Autodesk Inventor part; units mm, degrees
ref_plane "YZ Plane" through (0, 0, 0) normal (1, 0, 0) x (0, 1, 0)
ref_plane "XZ Plane" through (0, 0, 0) normal (0, 1, 0) x (-1, 0, 0)
ref_plane "XY Plane" through (0, 0, 0) normal (0, 0, 1) x (1, 0, 0)
sketch "Эскиз1" plane through (0, 0, 0) normal (0, 1, 0) x (-1, 0, 0)
  circle A0 centre (0, 0) radius 42
  line L0 (0, -42) -> (0, 42) construction
  circle A1 centre (18.0767, -25) radius 9
  circle A2 centre (-18.0767, -25) radius 9
  line L1 (39.598, -14) -> (-39.598, -14)
  circle A3 centre (0, -30.8507) radius 9
  circle A4 centre (0, 0) radius 30.8507 construction
  line L2 (0, 0) -> (12.9332, -39.9591) construction
  line L3 (0, 0) -> (-12.9332, -39.9591) construction
  line L4 (9.9159, -38.7553) -> (14.673, -37.2156)
  line L5 (14.673, -37.2156) -> (15.2888, -39.1184)
  line L6 (15.2888, -39.1184) -> (10.5318, -40.6581)
  line L7 (10.5318, -40.6581) -> (9.9159, -38.7553)
  line L8 (9.9159, -38.7553) -> (15.2888, -39.1184) construction
  line L9 (14.673, -37.2156) -> (10.5318, -40.6581) construction
  line L10 (-14.673, -37.2156) -> (-9.9159, -38.7553)
  line L11 (-9.9159, -38.7553) -> (-10.5318, -40.6581)
  line L12 (-10.5318, -40.6581) -> (-15.2888, -39.1184)
  line L13 (-15.2888, -39.1184) -> (-14.673, -37.2156)
  line L14 (-14.673, -37.2156) -> (-10.5318, -40.6581) construction
  line L15 (-9.9159, -38.7553) -> (-15.2888, -39.1184) construction
  line L16 (-2.5, -16.8507) -> (2.5, -16.8507)
  line L17 (2.5, -16.8507) -> (2.5, -18.8507)
  line L18 (2.5, -18.8507) -> (-2.5, -18.8507)
  line L19 (-2.5, -18.8507) -> (-2.5, -16.8507)
  line L20 (-2.5, -16.8507) -> (2.5, -18.8507) construction
  line L21 (2.5, -16.8507) -> (-2.5, -18.8507) construction
  circle A5 centre (0, 0) radius 17.0352
  circle A6 centre (0, -44.5) radius 2.5
  circle A7 centre (0, 0) radius 50
  circle A8 centre (0, -44.5) radius 4
  circle A9 centre (-32, -19) radius 2.5
  circle A10 centre (32, -19) radius 2.5
  circle A11 centre (0, 0) radius 44 construction
  circle A12 centre (0, 2) radius 44
  circle A13 centre (31.1127, -29.1127) radius 2.5
  circle A14 centre (-31.1127, -29.1127) radius 2.5
  point P0 (12.6024, -38.9369)
  point P1 (-12.6024, -38.9369)
  point P2 (0, -17.8507)
  point P3 (9.7056, -14)
  point P4 (2.5, -16.8507)
  point P5 (-9.7056, -14)
  point P6 (-15.2888, -39.1184)
  point P7 (10.5318, -40.6581)
  point P8 (-3.0315, -41.8904)
  point P9 (3.0315, -41.8904)
  point P10 (0, -42)
  point P11 (28.9734, -30.4063)
  point P12 (32.2615, -26.8923)
  point P13 (-32.2615, -26.8923)
  point P14 (-28.9734, -30.4063)
  dimension "d0" = 84
  dimension "d5" = 18
  dimension "d7" = 14
  dimension "d8" = 11
  dimension "d13" = 35.87
  dimension "d14" = 17.935
  dimension "d15" = 2
  dimension "d16" = 2
  dimension "d17" = 5
  dimension "d18" = 5
  dimension "d19" = 5
  dimension "d20" = 2
  dimension "d21" = 13
  dimension "d27" = 100
  dimension "d28" = 5
  dimension "d29" = 8
  dimension "d30" = 5
  dimension "d31" = 19
  dimension "d32" = 64
  dimension "d34" = 19
  dimension "d35" = 88
  dimension "d37" = 2
  dimension "d38" = 88
  dimension "d39" = 5
  dimension "d40" = 90
extrude "Выдавливание2" add sketch "Эскиз1" along normal blind 3 contours L1 A5 L19 L18 L17 A0 A13 L5 L4 L7 A8 L11 L10 L13 A14 | A8 A0 A12 | A12 A0 A8 | A8 A0
fillet "Сопряжение3" radius 6 2 edges at (39.598, 1.5, -14) (-39.598, 1.5, -14)
fillet "Сопряжение4" radius 5 2 edges at (-32.2615, 1.5, -26.8923) (-28.9734, 1.5, -30.4063)
fillet "Сопряжение5" radius 5 2 edges at (28.9734, 1.5, -30.4063) (32.2615, 1.5, -26.8923)
equation "\"d14\" = 0.5 * d13"
properties part number "Крепление АКБ" material "Пластик АБС"
Check sheet for the modelled part. Datum: model origin and axes. Units: mm. A direction names the side the tool comes from. Round coordinates to 2 decimals unless told otherwise and drop trailing zeros. Loops run counter-clockwise (first coordinate to the right, second up) from the corner with the lowest first, then second, coordinate; pieces in that order, holes last. Notation, with made-up numbers: M -33,-20 L 16,-20 A17 cw 16,-4 Z; hole C -22,31 d10. An arc over 180 degrees is marked long. One line per item, written item: value.
(1) Sectioned sample at B-B, the plane z = -35.5. Record the cut outline in (x, y), then the cut area to 3 significant figures.
Computed values:
outline: M -22.44,0 L -7.71,0 L -7.71,3 L -22.44,3 Z; M 7.71,0 L 22.44,0 L 22.44,3 L 7.71,3 Z
area: 88.4 mm^2
(2) Sectioned sample at A-A, the plane x = 0. Record the cut outline in (y, z).
Computed values:
outline: M 0,-42 L 3,-42 L 3,-39.85 L 0,-39.85 Z; M 0,-21.85 L 3,-21.85 L 3,-18.85 L 0,-18.85 Z
(3) Release check for a two-part mould opening along X. For faces 4 (the face through (0.5, 0, -21.6)), 5 (the face through (0, 1, -18.851)), 6 (the face through (29.3, 1.48, -27.39)) record: +X half, -X half, draft (parallel to the pull), parting line (faces both ways), or undercut.
Computed values:
face 4: draft
face 5: undercut
face 6: +X half
(4) Access from +Z, -Z, +X, -X, +Y, -Y to the whole of each face (thin tool, end or side, straight path). Record for faces 1 (the face through (10.22, 1.48, -39.69)), 2 (the face through (2.5, 1, -18)), 3 (the face through (14.985, 1.479, -38.18)).
Computed values:
face 1: +Y, -Y
face 2: +Z, +Y, -Y
face 3: -Z, +Y, -Y
(5) Thickness scan on line 1 (X direction, y = 0.65, z = -20.25); line 2 (X direction, y = 1.2, z = -22.75); line 3 (X direction, y = 2.4, z = -36.75). Record the ranges inside material, lowest first.
Computed values:
line 1: x = -35.93 to -34.17, -29.83 to -25.72, -10.43 to 10.43, 25.72 to 29.83, 34.17 to 35.93
line 2: x = -35.27 to -26.79, -9.36 to -3.92, 3.92 to 9.36, 26.79 to 35.27
line 3: x = -20.33 to -6.8, 6.8 to 20.33
(6) Sectioned sample at C-C, the plane y = 1.75. Count the separate pieces of the cut face and the enclosed holes in it, then the cut area to 3 significant figures.
Computed values:
separate pieces: 1
enclosed holes: 5
area: 681 mm^2
(7) Depth check by flat-ended pin: pin 1 Ø16 at (x, z) = (-18.08, -25) entering from +Y; pin 2 Ø1 at (y, z) = (2, -18) entering from +X. Enter the tip coordinate at first touch or a pass-through.
Computed values:
pin 1: passes through
pin 2: stops at x = 35.74
